from build123d import *

# Parameters (mm, degrees)
SKETCH_1_R          = 23
EXTRUDE_1_DEPTH     = 2
SKETCH_2_R          = 20
EXTRUDE_2_DEPTH     = 6
SKETCH_3_R          = 1.8
CUT_EXTRUDE_1_DEPTH = 34.496268449
SKETCH_4_R          = 10
CUT_EXTRUDE_2_DEPTH = 34.496268449
FILLET_1_R          = 1
CUT_EXTRUDE_5_DEPTH = 2.8
EXTRUDE_START       = -11
SKETCH_9_R          = 10
SKETCH_9_R_2        = 6.5
EXTRUDE_3_DEPTH     = 11
SKETCH_10_R         = 10
SKETCH_10_R_2       = 8.5
CUT_EXTRUDE_6_DEPTH = 3
FILLET_3_R          = 1.5
FILLET_4_R          = 5
SKETCH_11_R         = 8.5
CUT_EXTRUDE_7_DEPTH = 34.496268473


with BuildPart() as part:
    # 草图1 → 凸台-拉伸1 (new body)
    with BuildSketch(Plane.XY):
        Circle(SKETCH_1_R)
    extrude(amount=EXTRUDE_1_DEPTH)

    # 草图2 → 凸台-拉伸2 (add)
    with BuildSketch(Plane.XY.offset(2)):
        Circle(SKETCH_2_R)
    extrude(amount=EXTRUDE_2_DEPTH)

    # 草图3 → 切除-拉伸1 (cut, through all)
    with BuildSketch(Plane.XY.offset(8)):
        with Locations((0, 14)):
            Circle(SKETCH_3_R)
        with Locations((12.124355653, 7)):
            Circle(SKETCH_3_R)
        with Locations((12.124355653, -7)):
            Circle(SKETCH_3_R)
        with Locations((0, -14)):
            Circle(SKETCH_3_R)
        with Locations((-12.124355653, -7)):
            Circle(SKETCH_3_R)
        with Locations((-12.124355653, 7)):
            Circle(SKETCH_3_R)
    extrude(amount=-CUT_EXTRUDE_1_DEPTH, mode=Mode.SUBTRACT)

    # 草图4 → 切除-拉伸2 (cut, through all)
    with BuildSketch(Plane.XY.offset(8)):
        Circle(SKETCH_4_R)
    extrude(amount=-CUT_EXTRUDE_2_DEPTH, mode=Mode.SUBTRACT)

    # 圆角1
    fillet_1_edges = [part.edges().sort_by_distance(p)[0] for p in [
        (-20, 0, 8),
    ]]
    fillet(fillet_1_edges, radius=FILLET_1_R)

    # 草图8 → 切除-拉伸5 (cut)
    with BuildSketch(Plane(origin=(0, 0, 0), x_dir=(-1, 0, 0), z_dir=(0, 0, -1))):
        Polygon((-10.507774899, 9.8), (-13.740936407, 9.8), (-15.35751716, 7), (-13.740936407, 4.2), (-10.507774899, 4.2), (-8.891194146, 7), align=None)
        Polygon((3.233161507, 14), (1.616580754, 16.8), (-1.616580754, 16.8), (-3.233161507, 14), (-1.616580754, 11.2), (1.616580754, 11.2), align=None)
        Polygon((13.740936407, 4.2), (15.35751716, 7), (13.740936407, 9.8), (10.507774899, 9.8), (8.891194146, 7), (10.507774899, 4.2), align=None)
        Polygon((10.507774899, -9.8), (13.740936407, -9.8), (15.35751716, -7), (13.740936407, -4.2), (10.507774899, -4.2), (8.891194146, -7), align=None)
        Polygon((-3.233161507, -14), (-1.616580754, -16.8), (1.616580754, -16.8), (3.233161507, -14), (1.616580754, -11.2), (-1.616580754, -11.2), align=None)
        Polygon((-13.740936407, -4.2), (-15.35751716, -7), (-13.740936407, -9.8), (-10.507774899, -9.8), (-8.891194146, -7), (-10.507774899, -4.2), align=None)
    extrude(amount=-CUT_EXTRUDE_5_DEPTH, mode=Mode.SUBTRACT)

    # 草图9 → 凸台-拉伸3 (add)
    with BuildSketch(Plane(origin=(0, 0, 0), x_dir=(-1, 0, 0), z_dir=(0, 0, -1)).offset(EXTRUDE_START)):
        Circle(SKETCH_9_R)
        Circle(SKETCH_9_R_2, mode=Mode.SUBTRACT)
    extrude(amount=EXTRUDE_3_DEPTH)

    # 草图10 → 切除-拉伸6 (cut)
    with BuildSketch(Plane.XY.offset(11)):
        Circle(SKETCH_10_R)
        Circle(SKETCH_10_R_2, mode=Mode.SUBTRACT)
    extrude(amount=-CUT_EXTRUDE_6_DEPTH, mode=Mode.SUBTRACT)

    # 圆角3
    fillet_3_edges = [part.edges().sort_by_distance(p)[0] for p in [
        (-8.5, 0, 11),
    ]]
    fillet(fillet_3_edges, radius=FILLET_3_R)

    # 圆角4
    # the kernel refuses this fillet: 5 mm, written as the material it takes off along each edge
    with BuildSketch(Plane(origin=(0, 0, 0), x_dir=(-1, 0, 0), z_dir=(0, -1, 0))) as fillet_4_piece_1:
        with BuildLine():
            CenterArc((6.5 + FILLET_4_R, -FILLET_4_R), FILLET_4_R, 90, 90)
            Line((6.5 + FILLET_4_R, 0), (6.5, 0))
            Line((6.5, 0), (6.5, -FILLET_4_R))
        make_face()
    revolve(axis=Axis((0, 0, 0), (0, 0, -1)), mode=Mode.SUBTRACT)

    # 草图11 → 切除-拉伸7 (cut, through all)
    with BuildSketch(Plane.XY.offset(8)):
        Circle(SKETCH_11_R)
    extrude(amount=CUT_EXTRUDE_7_DEPTH, mode=Mode.SUBTRACT)


solid = part.part
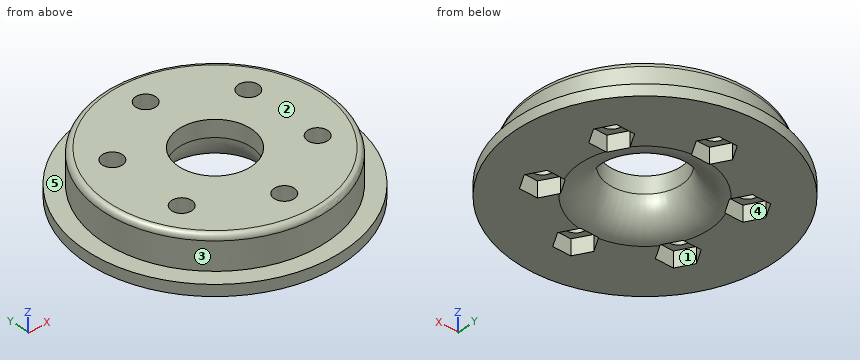
Read the model definition and answer for the solid it produces. Units are mm, in the model's axes. Face numbers are marked on the shaded views. A direction names the side the tool comes from. Round coordinates to 2 decimals unless told otherwise and drop trailing zeros. Write each loop counter-clockwise with the first axis right and the second up, starting at its lowest first coordinate (ties: lowest second). Pieces come first, ordered by that corner, then holes.
1. The part is cut by section A-A, the plane y = 0. Determine the outline of the cut face in (x, z).
2. Straight lines are drawn through the part: L1, parallel to Y at x = 0, z = 6; L2, parallel to Y at x = 0.5, z = 5.75; L3, parallel to Y at x = 13, z = 3.25. For each, find the intervals that lie inside material, in ascending order.
3. Which of the six approach directions +Z, -Z, +X, -X, +Y, -Y give full straight-line access (tool end or side, diameter ignored) to the marked faces 1 and 2?
4. Given pin 1 Ø1.7 at (x, y) = (11, 6.5) entering from -Z; pin 2 Ø0.8 at (x, z) = (-0.5, 1) entering from -Y; pin 3 Ø3 at (y, z) = (-6.5, 5.5) entering from -X, each flat-ended and moving along its own axis, determine where each tip first touches the part or whether it passes through.
5. The part is cut by section B-B, the plane z = 5.75. Determine the outline of the cut face in (x, y).
6. Determine the mould class of the marked faces 3, 4 and 5 for opening direction X: pulls with the +X half, pulls with the -X half, needs draft (parallel to the pull), parting line crosses it, or undercut.
7. The part is cut by section C-C, the plane x = 0. State how many separate pieces and enclosed holes the cut face has, then the cut area to 3 significant figures.
Values:
1. outline: (-23, 0) - (-11.5, 0) arc R5 ccw to (-6.5, 5) - (-6.5, 8) - (-19, 8) arc R1 ccw to (-20, 7) - (-20, 2) - (-23, 2) - close; (6.5, 5) arc R5 ccw to (11.5, 0) - (23, 0) - (23, 2) - (20, 2) - (20, 7) arc R1 ccw to (19, 8) - (6.5, 8) - close
2. L1: y = -20 to -15.8, -12.2 to -6.5, 6.5 to 12.2, 15.8 to 20
2. L2: y = -19.99 to -15.73, -12.27 to -6.48, 6.48 to 12.27, 15.73 to 19.99
2. L3: y = -15.2 to -8.57, -5.43 to 5.43, 8.57 to 15.2
3. face 1: -Z
3. face 2: +Z, +X, -X, +Y, -Y
4. pin 1: stops at z = 2.8
4. pin 2: stops at y = -23
4. pin 3: stops at x = -19.36
5. outline: circle Ø40 at (0, 0); hole circle Ø3.6 at (-12.12, -7); hole circle Ø3.6 at (-12.12, 7); hole circle Ø13 at (0, 0); hole circle Ø3.6 at (0, -14); hole circle Ø3.6 at (0, 14); hole circle Ø3.6 at (12.12, -7); hole circle Ø3.6 at (12.12, 7)
6. face 3: parting line crosses it
6. face 4: undercut
6. face 5: needs draft
7. separate pieces: 4
7. enclosed holes: 0
7. area: 148 mm2
